Geometry: final body of the model. Coordinates: model frame, mm. Face numbers are marked on the shaded views. A direction names the side the tool comes from. Give positions to 0.01 mm unless a question says otherwise; leave off trailing zeros. Loops run counter-clockwise (first coordinate to the right, second up) from the corner with the lowest first, then second, coordinate; pieces in that order, holes last. Notation, with made-up numbers: (-40, -21.5) -> (-23, -21.5) arc R28 cw to (-23, 3.5) -> close; hole circle Ø11 at (-39, 83.25). An arc over 180 degrees is marked (long way). Answer in a Markdown table with one row per item. Add a question column.
from build123d import *

# Parameters (mm, degrees)
SKETCH1_W           = 20
SKETCH1_H           = 10
BOSS_EXTRUDE1_DEPTH = 12
SKETCH2_W           = 8
SKETCH2_H           = 10
CUT_EXTRUDE1_DEPTH  = 8
FILLET1_R           = 4
SKETCH3_R           = 1.75
CUT_EXTRUDE2_DEPTH  = 21
FILLET2_R           = 3
SKETCH5_R           = 4
BOSS_EXTRUDE2_DEPTH = 9
SKETCH6_R           = 2
CUT_EXTRUDE3_DEPTH  = 7


with BuildPart() as part:
    # Sketch1 → Boss-Extrude1 (new body)
    with BuildSketch(Plane(origin=(0, 0, 0), x_dir=(1, 0, 0), z_dir=(0, 1, 0))):
        Rectangle(SKETCH1_W, SKETCH1_H)
    extrude(amount=BOSS_EXTRUDE1_DEPTH)

    # Sketch2 → Cut-Extrude1 (cut)
    with BuildSketch(Plane(origin=(0, 12, 0), x_dir=(1, 0, 0), z_dir=(0, 1, 0))):
        Rectangle(SKETCH2_W, SKETCH2_H)
    extrude(amount=-CUT_EXTRUDE1_DEPTH, mode=Mode.SUBTRACT)

    # Fillet1
    fillet1_edges = [part.edges().sort_by_distance(p)[0] for p in [
        (-7, 12, -5),
        (7, 12, 5),
        (-7, 12, 5),
        (7, 12, -5),
    ]]
    fillet(fillet1_edges, radius=FILLET1_R)

    # Sketch3 → Cut-Extrude2 (cut, through all)
    with BuildSketch(Plane.ZY.offset(10)):
        with Locations((0, 8)):
            Circle(SKETCH3_R)
    extrude(amount=-CUT_EXTRUDE2_DEPTH, mode=Mode.SUBTRACT)

    # Fillet2
    fillet2_edges = [part.edges().sort_by_distance(p)[0] for p in [
        (-10, 0, 0),
        (10, 0, 0),
    ]]
    fillet(fillet2_edges, radius=FILLET2_R)

    # Sketch5 → Boss-Extrude2 (add)
    with BuildSketch(Plane.XZ):
        Circle(SKETCH5_R)
    extrude(amount=BOSS_EXTRUDE2_DEPTH)

    # Sketch6 → Cut-Extrude3 (cut)
    with BuildSketch(Plane.XZ.offset(9)):
        Circle(SKETCH6_R)
    extrude(amount=-CUT_EXTRUDE3_DEPTH, mode=Mode.SUBTRACT)


solid = part.part
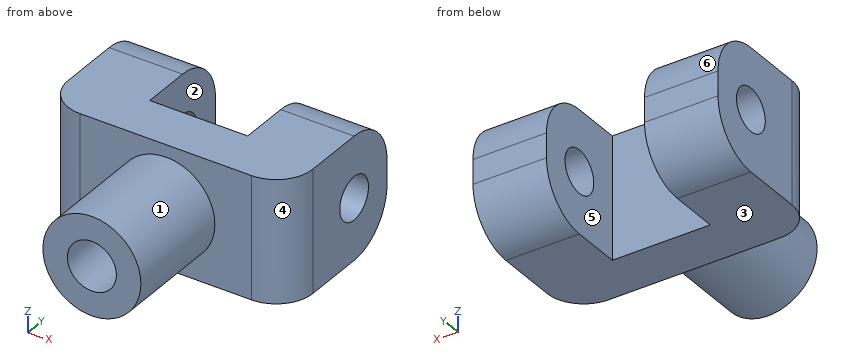
(1) Cut plane D-D on x = 0. Return the cut outline in (y, z).
(2) Cut plane B-B on x = -5.25. Return the cut outline in (y, z), then the cut area to 3 significant figures.
(3) Reachability of the marked faces 1, 2 and 3 from +Z, -Z, +X, -X, +Y, -Y: full face, straight path, thin tool, end or side. Return the list, or none.
(4) Pin query (flat end, axial travel): pin 1 Ø12 at (x, y) = (-1.5, -0.5) entering from -Z; pin 2 Ø4.5 at (x, z) = (0, 0) entering from +Y; pin 3 Ø1 at (x, y) = (-2.5, -3) entering from +Z; pin 4 Ø2 at (y, z) = (-0.5, -0.5) entering from -X. Return the tip coordinate at first contact, or that it passes through.
(5) Cut plane A-A on z = 0. Return the cut outline in (x, y), then the cut area to 3 significant figures.
(6) Cut plane C-C on y = -4.5. Return the cut outline in (x, z).
(7) Material intervals for line 1 along X through (y, z) = (6, -2.25); line 2 along Y through (x, z) = (-6.35, 0); line 3 along Y through (x, z) = (-1.5, -4.25), sorted ascending. Write a range as from..to.
(8) Draft query along X for the marked faces 4, 5 and 6. Return one class per face: +X half, -X half, draft (parallel to the pull), parting line (faces both ways), or undercut.
Answer list:
| question | item | result |
|---|---|---|
| 1 | outline | (-9, -4) -> (0, -4) -> (0, -5) -> (4, -5) -> (4, 5) -> (0, 5) -> (0, 4) -> (-9, 4) -> (-9, 2) -> (-2, 2) -> (-2, -2) -> (-9, -2) -> close |
| 2 | outline | (0, -5) -> (8, -5) arc R4 ccw to (12, -1) -> (12, 1) arc R4 ccw to (8, 5) -> (0, 5) -> close; hole circle Ø3.5 at (8, 0) |
| 2 | area | 104 mm² |
| 3 | face 1 | -Y |
| 3 | face 2 | +Z, -Z, +Y |
| 3 | face 3 | -Z, +X, -X, +Y, -Y |
| 4 | pin 1 | stops at z = -5 |
| 4 | pin 2 | stops at y = 4 |
| 4 | pin 3 | stops at z = 3.46 |
| 4 | pin 4 | stops at x = -8.66 |
| 5 | outline | (-10, 3) arc R3 ccw to (-7, 0) -> (-4, 0) -> (-4, -9) -> (-2, -9) -> (-2, -2) -> (2, -2) -> (2, -9) -> (4, -9) -> (4, 0) -> (7, 0) arc R3 ccw to (10, 3) -> (10, 6.25) -> (4, 6.25) -> (4, 4) -> (-4, 4) -> (-4, 6.25) -> (-10, 6.25) -> close; (-10, 9.75) -> (-4, 9.75) -> (-4, 12) -> (-10, 12) -> close; (4, 9.75) -> (10, 9.75) -> (10, 12) -> (4, 12) -> close |
| 5 | area | 174 mm² |
| 6 | outline | circle Ø8 at (0, 0); hole circle Ø4 at (0, 0) |
| 7 | line 1 | x = -10..-4, 4..10 |
| 7 | line 2 | y = 0..6.25, 9.75..12 |
| 7 | line 3 | y = 0..4 |
| 8 | face 4 | +X half |
| 8 | face 5 | undercut |
| 8 | face 6 | draft |
